```python
from build123d import *

# Parameters (mm, degrees)
SKETCH1_W              = 48
SKETCH1_H              = 17.5
BODY_DEPTH             = 30
TUBE_CUTOUT_DEPTH      = 40.402569713
SKETCH3_R              = 2.625
CUT_EXTRUDE_M5_DEPTH   = 43.216702856
SLOPE_DEPTH            = 40.402569713
BOLT_HEAD_CUTOUT_START = -6.5
SKETCH5_R              = 4.75
BOLT_HEAD_CUTOUT_DEPTH = 23
FILLET_2_R             = 10
SKETCH7_W              = 48
SKETCH7_H              = 30
CLEARANCE_DEPTH        = 0.2


with BuildPart() as part:
    # Sketch1 → body (new body)
    with BuildSketch(Plane.XY):
        Rectangle(SKETCH1_W, SKETCH1_H)
    extrude(amount=BODY_DEPTH)

    # Sketch2 → tube_cutout (cut, through all)
    with BuildSketch(Plane.XY):
        with BuildLine():
            Line((13.125, -8.75), (-13.125, -8.75))
            ThreePointArc((-13.125, -8.75), (0, 4.375), (13.125, -8.75))
        make_face()
    extrude(amount=TUBE_CUTOUT_DEPTH, mode=Mode.SUBTRACT)

    # Sketch3 → Cut-Extrude M5 (cut, through all)
    with BuildSketch(Plane.XZ.offset(8.75)):
        with Locations(Location((18.5625, 22.5, 0), (0, 0, 270))):
            Circle(SKETCH3_R)
        with Locations(Location((18.5625, 7.5, 0), (0, 0, 270))):
            Circle(SKETCH3_R)
        with Locations(Location((-18.5625, 7.5, 0), (0, 0, 90))):
            Circle(SKETCH3_R)
        with Locations(Location((-18.5625, 22.5, 0), (0, 0, 90))):
            Circle(SKETCH3_R)
    extrude(amount=-CUT_EXTRUDE_M5_DEPTH, mode=Mode.SUBTRACT)

    # Sketch4 → slope (cut, through all)
    with BuildSketch(Plane.XY):
        Polygon((-24, 8.75), (-24, -3.25), (-12, 8.75), align=None)
        Polygon((24, -3.25), (12, 8.75), (24, 8.75), align=None)
    extrude(amount=SLOPE_DEPTH, mode=Mode.SUBTRACT)

    # Sketch5 → bolt_head_cutout (cut)
    with BuildSketch(Plane.XZ.offset(8.75).offset(BOLT_HEAD_CUTOUT_START)):
        with Locations((18.5625, 22.5)):
            Circle(SKETCH5_R)
        with Locations((18.5625, 7.5)):
            Circle(SKETCH5_R)
        with Locations((-18.5625, 7.5)):
            Circle(SKETCH5_R)
        with Locations((-18.5625, 22.5)):
            Circle(SKETCH5_R)
    extrude(amount=-BOLT_HEAD_CUTOUT_DEPTH, mode=Mode.SUBTRACT)

    # fillet 2
    # the kernel refuses this fillet: 10 mm, written as the material it takes off along each edge
    with BuildSketch(Plane(origin=(24, -3.25, -10.355339059), x_dir=(-0.7071067811865475, 0.7071067811865478, 0), z_dir=(0, 0, 1)), Plane(origin=(12, 8.75, -10.355339059), x_dir=(-1, 0, 0), z_dir=(0, 0, 1)), Plane(origin=(-12, 8.75, -10.355339059), x_dir=(-0.7071067811865474, -0.7071067811865478, 0), z_dir=(0, 0, 1))) as fillet_2_piece_1:
        with BuildLine():
            CenterArc((FILLET_2_R * 0.414213562373, FILLET_2_R), FILLET_2_R, 225, 45)
            Line((-FILLET_2_R * 0.292893218813, FILLET_2_R * 0.292893218813), (0, 0))
            Line((0, 0), (FILLET_2_R * 0.414213562373, 0))
        make_face()
    extrude(amount=50.710678119, mode=Mode.SUBTRACT)
    with BuildSketch(Plane(origin=(-24, -3.25, -10.355339059), x_dir=(0.7071067811865469, 0.707106781186548, 0), z_dir=(0, 0, 1))) as fillet_2_piece_2:
        with BuildLine():
            CenterArc((FILLET_2_R * 0.414213562373, -FILLET_2_R), FILLET_2_R, 90, 45)
            Line((-FILLET_2_R * 0.292893218813, -FILLET_2_R * 0.292893218813), (0, 0))
            Line((0, 0), (FILLET_2_R * 0.414213562373, 0))
        make_face()
    extrude(amount=50.710678119, mode=Mode.SUBTRACT)

    # Sketch7 → clearance (cut)
    with BuildSketch(Plane.XZ.offset(8.75)):
        with Locations((0, 15)):
            Rectangle(SKETCH7_W, SKETCH7_H)
    extrude(amount=-CLEARANCE_DEPTH, mode=Mode.SUBTRACT)


solid = part.part
```
Input: part model. Units: mm. Frame: model coordinates. A direction names the side the tool comes from. Give positions to 0.01 mm unless a question says otherwise; leave off trailing zeros. Order: outer loops, then holes, each group sorted by start corner. A loop starts at its lowest first (then second) coordinate and runs counter-clockwise, first axis right, second up. Notation, with made-up numbers: M 5.5,-22.5 L 9.5,-22.5 A35 ccw 9.5,16.5 Z; hole C -39.5,36 d2. An arc over 180 degrees is marked long. One line per question, with ' | ' between items. Start each with the question number.
1. Section query A-A (z = 22.5). Count the separate pieces of the cut face and the enclosed holes in it, and give its area (3 significant figures).
2. Access query for faces 4 (the face through (13.816, 1.2, 7.671)), 5 (the face through (11.735, 7.968, 14.79)). Directions: +Z, -Z, +X, -X, +Y, -Y. A direction counts if a zero-diameter tool reaches every point of the face in a straight line with its end or side. Return the directions, or none.
3. Material intervals for probe 1 along X at (y, z) = (-6.5, 7.5); probe 2 along Z at (x, y) = (-16.5, -0.5); probe 3 along X at (y, z) = (-4.25, 22.5), sorted ascending. Write a range as [from, to].
4. Section query B-B (y = -1). Return the cut outline in (x, z).
5. First-contact query: pin 1 Ø11 at (x, z) = (-18.56, 7.5) entering from +Y; pin 2 Ø15 at (x, z) = (18.56, 22.5) entering from +Y; pin 3 Ø1 at (x, z) = (-4.5, 17) entering from -Y. Flat tips, straight axial feed; report the tip coordinate or a pass-through.
6. Section query C-C (z = 17). Return the cut outline in (x, y) (3 decimals).
7. Pull-direction query (Z, two-part tool) for faces 1 (the face through (0, 6, 30)), 2 (the face through (0, 8.75, 15)), 3 (the face through (-20.34, -5.44, 20.57)); classes: released by +Z, released by -Z, zero draft, split by the parting line, or undercut.
Here are the results:
1) separate pieces: 3 | enclosed holes: 0 | area: 263 mm²
2) face 4: +Y | face 5: +Z, -Z, +X, +Y
3) probe 1: [-23.96, -21.19], [-15.94, -12.93], [12.93, 15.94], [21.19, 23.96] | probe 2: [0, 3.22], [11.78, 18.22], [26.78, 30] | probe 3: [-23.49, -21.19], [-15.94, -12.33], [12.33, 15.94], [21.19, 23.49]
4) outline: M -21.69,0 L -10.59,0 L -10.59,30 L -21.69,30 L -21.69,26.07 A4.75 cw long -21.69,18.93 L -21.69,11.07 A4.75 cw long -21.69,3.93 Z; M 10.59,0 L 21.69,0 L 21.69,3.93 A4.75 cw long 21.69,11.07 L 21.69,18.93 A4.75 cw long 21.69,26.07 L 21.69,30 L 10.59,30 Z
5) pin 1: y = 7.29 | pin 2: y = 8.22 | pin 3: y = 3.39
6) outline: M -24,-8.55 L -13.123,-8.55 A13.125 cw 13.123,-8.55 L 24,-8.55 L 24,-7.392 A10 ccw 21.071,-0.321 L 14.929,5.821 A10 ccw 7.858,8.75 L -7.858,8.75 A10 ccw -14.929,5.821 L -21.071,-0.321 A10 ccw -24,-7.392 Z
7) face 1: released by +Z | face 2: zero draft | face 3: undercut
